Work out the finished part from the listing and answer in its coordinate system (mm). A direction names the side the tool comes from. Round coordinates to 2 decimals unless told otherwise and drop trailing zeros. Order: outer loops, then holes, each group sorted by start corner. A loop starts at its lowest first (then second) coordinate and runs counter-clockwise, first axis right, second up. Notation, with made-up numbers: (71.25, 66) - (92.25, 66) arc R17 cw to (92.25, 97) - close; hole circle Ø5 at (-7, 46). An arc over 180 degrees is marked (long way). Put each result on its own line as item: value.
```python
from build123d import *

# Parameters (mm, degrees)
EXTRUDE_2_DEPTH   = 5
EXTRUDE_3_DEPTH   = 3.8
EXTRUDE_4_DEPTH   = 1
CHAMFER_1_SIZE    = 2
HOLE_WIZARD_M31_D = 3.4


with BuildPart() as part:
    # Эскиз2 → Бобышка-Вытянуть2 (new body)
    with BuildSketch(Plane(origin=(0, 0, 0), x_dir=(1, 0, 0), z_dir=(0, 1, 0))):
        Polygon((-21.75, 7), (-21.75, -7), (-21.75, -11.7), (-21.75, -22.7), (21.75, -22.7), (21.75, 22.7), (-21.75, 22.7), (-21.75, 11.7), align=None)
        Polygon((-16.75, 17.7), (16.75, 17.7), (16.75, -17.7), (-16.75, -17.7), (-16.75, -11.7), (-16.75, -7), (-16.75, 7), (-16.75, 11.7), align=None, mode=Mode.SUBTRACT)
    extrude(amount=EXTRUDE_2_DEPTH)

    # Эскиз3 → Бобышка-Вытянуть3 (add)
    with BuildSketch(Plane(origin=(0, 5, 0), x_dir=(1, 0, 0), z_dir=(0, 1, 0))):
        with BuildLine():
            Line((-16.75, 17.7), (-16.75, 12.7))
            Line((-16.75, 12.7), (-15.75, 12.7))
            Line((-15.75, 12.7), (-13.001919935, 12.7))
            ThreePointArc((-13.001919935, 12.7), (-12.294813154, 12.992893219), (-12.001919935, 13.7))
            Line((-12.001919935, 13.7), (-12.001919935, 16.7))
            Line((-12.001919935, 16.7), (-12.001919935, 17.7))
            Line((-12.001919935, 17.7), (-16.75, 17.7))
        make_face()
        with BuildLine():
            Line((15.75, 12.7), (16.75, 12.7))
            Line((16.75, 12.7), (16.75, 17.7))
            Line((16.75, 17.7), (11.75, 17.7))
            Line((11.75, 17.7), (11.75, 16.7))
            Line((11.75, 16.7), (11.75, 13.7))
            ThreePointArc((11.75, 13.7), (12.042893219, 12.992893219), (12.75, 12.7))
            Line((12.75, 12.7), (15.75, 12.7))
        make_face()
        with BuildLine():
            Line((11.75, -16.7), (11.75, -17.7))
            Line((11.75, -17.7), (16.75, -17.7))
            Line((16.75, -17.7), (16.75, -12.7))
            Line((16.75, -12.7), (15.75, -12.7))
            Line((15.75, -12.7), (12.75, -12.7))
            ThreePointArc((12.75, -12.7), (12.042893219, -12.992893219), (11.75, -13.7))
            Line((11.75, -13.7), (11.75, -16.7))
        make_face()
        with BuildLine():
            Line((-12.001919935, -16.7), (-12.001919935, -13.7))
            ThreePointArc((-12.001919935, -13.7), (-12.294813154, -12.992893219), (-13.001919935, -12.7))
            Line((-13.001919935, -12.7), (-15.75, -12.7))
            Line((-15.75, -12.7), (-16.75, -12.7))
            Line((-16.75, -12.7), (-16.75, -17.7))
            Line((-16.75, -17.7), (-12.001919935, -17.7))
            Line((-12.001919935, -17.7), (-12.001919935, -16.7))
        make_face()
    extrude(amount=-EXTRUDE_3_DEPTH)

    # Эскиз4 → Бобышка-Вытянуть4 (add)
    with BuildSketch(Plane(origin=(0, 5, 0), x_dir=(1, 0, 0), z_dir=(0, 1, 0))):
        with BuildLine():
            Line((-16.75, -12.7), (-13.001919935, -12.7))
            ThreePointArc((-13.001919935, -12.7), (-12.294813154, -12.992893219), (-12.001919935, -13.7))
            Line((-12.001919935, -13.7), (-12.001919935, -17.7))
            Line((-12.001919935, -17.7), (11.75, -17.7))
            Line((11.75, -17.7), (11.75, -13.7))
            ThreePointArc((11.75, -13.7), (12.042893219, -12.992893219), (12.75, -12.7))
            Line((12.75, -12.7), (16.75, -12.7))
            Line((16.75, -12.7), (16.75, 12.7))
            Line((16.75, 12.7), (12.75, 12.7))
            ThreePointArc((12.75, 12.7), (12.042893219, 12.992893219), (11.75, 13.7))
            Line((11.75, 13.7), (11.75, 17.7))
            Line((11.75, 17.7), (-12.001919935, 17.7))
            Line((-12.001919935, 17.7), (-12.001919935, 13.7))
            ThreePointArc((-12.001919935, 13.7), (-12.294813154, 12.992893219), (-13.001919935, 12.7))
            Line((-13.001919935, 12.7), (-16.75, 12.7))
            Line((-16.75, 12.7), (-16.75, -12.7))
        make_face()
        with BuildLine():
            Line((-4.8, -15.71), (8.9, -15.71))
            ThreePointArc((8.9, -15.71), (9.960660172, -15.270660172), (10.4, -14.21))
            Line((10.4, -14.21), (10.4, 14.21))
            ThreePointArc((10.4, 14.21), (9.960660172, 15.270660172), (8.9, 15.71))
            Line((8.9, 15.71), (-4.8, 15.71))
            ThreePointArc((-4.8, 15.71), (-5.860660172, 15.270660172), (-6.3, 14.21))
            Line((-6.3, 14.21), (-6.3, -14.21))
            ThreePointArc((-6.3, -14.21), (-5.860660172, -15.270660172), (-4.8, -15.71))
        make_face(mode=Mode.SUBTRACT)
    extrude(amount=-EXTRUDE_4_DEPTH)

    # Фаска1
    chamfer_1_edges = [part.edges().sort_by_distance(p)[0] for p in [
        (-21.75, 2.5, -22.7),
        (21.75, 2.5, -22.7),
        (21.75, 2.5, 22.7),
        (-21.75, 2.5, 22.7),
        (-21.75, 5, 0),
        (0, 5, 22.7),
        (21.75, 5, 0),
        (0, 5, -22.7),
    ]]
    chamfer(chamfer_1_edges, length=CHAMFER_1_SIZE)

    # Отверстие с зазором M31 (through all)
    with Locations(Plane(origin=(0, 5, 0), x_dir=(1, 0, 0), z_dir=(0, 1, 0))):
        with Locations((14.25, -15.2), (14.25, 15.2), (-14.375959967, 15.2), (-14.375959967, -15.2)):
            Hole(HOLE_WIZARD_M31_D / 2)


solid = part.part
```
1) A cutting plane is placed at D-D on z = -15.2. Write down the section's boundary in (x, y), then the cut area to 3 significant figures.
Findings below:
outline: (-21.75, 0) - (-16.75, 0) - (-16.75, 1.2) - (-16.08, 1.2) - (-16.08, 5) - (-19.75, 5) - (-21.75, 3) - close; (-12.68, 1.2) - (-12, 1.2) - (-12, 4) - (-5.93, 4) - (-5.93, 5) - (-12.68, 5) - close; (10.03, 4) - (11.75, 4) - (11.75, 1.2) - (12.55, 1.2) - (12.55, 5) - (10.03, 5) - close; (15.95, 1.2) - (16.75, 1.2) - (16.75, 0) - (21.75, 0) - (21.75, 3) - (19.75, 5) - (15.95, 5) - close
area: 65.0 mm2
2) A cutting plane is placed at C-C on x = -4. Write down the section's boundary in (y, z), then the cut area to 3 significant figures.
Findings below:
outline: (0, -22.7) - (3, -22.7) - (5, -20.7) - (5, -15.71) - (4, -15.71) - (4, -17.7) - (0, -17.7) - close; (0, 17.7) - (4, 17.7) - (4, 15.71) - (5, 15.71) - (5, 20.7) - (3, 22.7) - (0, 22.7) - close
area: 50.0 mm2
3) Given pin 1 Ø3 at (x, z) = (14.25, 15.2) entering from -Y; pin 2 Ø12 at (x, z) = (10, -5) entering from -Y; pin 3 Ø1.4 at (y, z) = (3.5, 15) entering from -X; pin 4 Ø4 at (x, z) = (-14.38, -15.2) entering from -Y, each flat-ended and moving along its own axis, determine where each tip first touches the part or whether it passes through.
Findings below:
pin 1: passes through
pin 2: stops at y = 4
pin 3: stops at x = -21.75
pin 4: stops at y = 1.2
4) Straight lines are drawn through the part: L1, parallel to X at y = 2.7, z = 15.2; L2, parallel to Z at x = 14.25, y = 2.85; L3, parallel to X at y = 2.25, z = -9.5. For each, find the intervals that lie inside material, in ascending order. Write a range as from..to.
Findings below:
L1: x = -21.75..-16.08, -12.68..-12, 11.75..12.55, 15.95..21.75
L2: z = -22.7..-16.9, -13.5..-12.7, 12.7..13.5, 16.9..22.7
L3: x = -21.75..-16.75, 16.75..21.75
5) For a pull along Z with two mould halves and no side action, classify faces 4 (the flat face through (-20.76, 3.99, -0.29)), 5 (the flat face through (-15, 3, -12.7)), 6 (the flat face through (-0.3, 4, 21.7)) as pulls with the +Z half, pulls with the -Z half, needs draft (parallel to the pull), parting line crosses it, or undercut.
Findings below:
face 4: needs draft
face 5: undercut
face 6: pulls with the +Z half
6) A cutting plane is placed at B-B on z = -7.5. Write down the section's boundary in (x, y).
Findings below:
outline: (-21.75, 0) - (-16.75, 0) - (-16.75, 4) - (-6.3, 4) - (-6.3, 5) - (-19.75, 5) - (-21.75, 3) - close; (10.4, 4) - (16.75, 4) - (16.75, 0) - (21.75, 0) - (21.75, 3) - (19.75, 5) - (10.4, 5) - close
7) A cutting plane is placed at A-A on x = 14.25. Write down the section's boundary in (y, z), then the cut area to 3 significant figures.
Findings below:
outline: (0, -22.7) - (3, -22.7) - (5, -20.7) - (5, -16.9) - (1.2, -16.9) - (1.2, -17.7) - (0, -17.7) - close; (0, 17.7) - (1.2, 17.7) - (1.2, 16.9) - (5, 16.9) - (5, 20.7) - (3, 22.7) - (0, 22.7) - close; (1.2, -13.5) - (5, -13.5) - (5, 13.5) - (1.2, 13.5) - (1.2, 12.7) - (4, 12.7) - (4, -12.7) - (1.2, -12.7) - close
area: 83.6 mm2
8) For faces 1 (the flat face through (2, 4.5, 15.71)), 2 (the flat face through (0.3, 4, -21.7)), 3 (the flat face through (-15, 3, 12.7)), determine the directions among +Z, -Z, +X, -X, +Y, -Y from which every point of the face is accessible in a straight line to the end or side of a thin tool.
Findings below:
face 1: +Y, -Y
face 2: -Z, +X, -X, +Y
face 3: -Y
